Can you work these out from the model? Positions are in its coordinate system, mm. A direction names the side the tool comes from. Round coordinates to 2 decimals unless told otherwise and drop trailing zeros. Write each loop counter-clockwise with the first axis right and the second up, starting at its lowest first coordinate (ties: lowest second). Pieces come first, ordered by that corner, then holes. Notation, with made-up numbers: M 89.25,-34 L 103.25,-34 A17 ccw 103.25,-30 Z; hole C 45,36 d6. An arc over 180 degrees is marked long. Answer as a JSON object with one key per item and string values. Group by question number.
1) Please list where these lines run through material, in increasing order: L1, parallel to X at y = 14.75, z = 31; L2, parallel to X at y = 10.5, z = 2; L3, parallel to Z at x = -3, y = 12. Write a range as [from, to].
2) On a 3-axis mill with a long thin cutter (end or side, diameter ignored), from which of +Z, -Z, +X, -X, +Y, -Y can I reach the whole of each face in a straight line? I mean faces 4 (the flat face through (-4, 12, -37.5)), 5 (the flat face through (0, 13, 13.5)), 6 (the flat face through (-2, 13, 30)), 7 (the flat face through (3, 13, -31)). Say none if no direction works.
3) Suppose I cut it at A-A, the plane z = -29. Write out the boundary of the cut face in (x, y), and give its area (3 significant figures).
4) If we mould it in two halves opening along X, with no side actions, what happens to faces 1 (the flat face through (6, 12, 37.5)), 2 (the flat face through (9, 12, 1)), 3 (the flat face through (3, 13, 31))? For each: +X half, -X half, draft (parallel to the pull), parting line (faces both ways), or undercut.
5) Suppose I cut it at D-D, the plane y = 12.5. State how many separate pieces and enclosed holes the cut face has, and give its area (3 significant figures).
6) Suppose I cut it at C-C, the plane x = 4.25. Write out the boundary of the cut face in (y, z), and give its area (3 significant figures).
7) Suppose I cut it at B-B, the plane y = 9.5. Write out the boundary of the cut face in (x, z) (3 decimals), and give its area (3 significant figures).
8) I'm going to push flat-ended pins straight in: pin 1 Ø1.8 at (y, z) = (12.5, 32.62) entering from -X; pin 2 Ø3 at (y, z) = (6.5, -32.5) entering from -X; pin 3 Ø8.5 at (y, z) = (14, -31.5) entering from -X. Where does each tip first touch, or does it pass through?
Autodesk Inventor part; units mm, degrees
ref_plane "YZ Plane" through (0, 0, 0) normal (1, 0, 0) x (0, 1, 0)
ref_plane "XZ Plane" through (0, 0, 0) normal (0, 1, 0) x (-1, 0, 0)
ref_plane "XY Plane" through (0, 0, 0) normal (0, 0, 1) x (1, 0, 0)
sketch "Boceto2" plane through (0, 0, 0) normal (0, 1, 0) x (-1, 0, 0)
  line L0 (-10, 37.5) -> (10, 37.5)
  line L1 (10, 37.5) -> (10, -37.5)
  line L2 (10, -37.5) -> (-10, -37.5)
  line L3 (-10, -37.5) -> (-10, 37.5)
  line L4 (-10, 37.5) -> (10, -37.5) construction
  line L5 (10, 37.5) -> (-10, -37.5) construction
  point P0 (0, 0)
  dimension "d10" = 20
  dimension "d11" = 75
extrude "Extrusión1" add sketch "Boceto2" along normal blind 25
sketch "Boceto3" plane through (0, 25, 0) normal (0, 1, 0) x (1, 0, 0)
  line L0 (-10, -37.5) -> (10, -37.5)
  line L1 (10, -37.5) -> (10, 37.5)
  line L2 (10, 37.5) -> (-10, 37.5)
  line L3 (-10, 37.5) -> (-10, -37.5)
  arc A0 (3, -26.6962) -> (-2, -27.1569) centre (0, -21.5) ccw
  arc A1 (-8, -21.5) -> (-5, -27.745) centre (0, -21.5) ccw
  line L4 (-10, -37.5) -> (10, -37.5)
  line L5 (3, -37.5) -> (-2, -37.5)
  line L6 (3, -26.6962) -> (3, -37.5)
  line L7 (-5, -37.5) -> (-5, -27.745)
  line L8 (-8, -21.5) -> (-8, 21.5)
  line L9 (-5, -13.5) -> (5, -13.5)
  line L10 (-5, -13.5) -> (-5, 13.5)
  line L11 (7, 0) -> (10, 0)
  line L12 (-2, -37.5) -> (-2, -27.1569)
  line L13 (10, 0) -> (7, 0)
  arc A2 (-2, 27.1569) -> (3, 26.6962) centre (0, 21.5) ccw
  arc A3 (-5, 27.745) -> (-8, 21.5) centre (0, 21.5) ccw
  line L14 (3, 37.5) -> (-2, 37.5)
  line L15 (3, 26.6962) -> (3, 37.5)
  line L16 (-5, 37.5) -> (-5, 27.745)
  line L17 (-8, 21.5) -> (-8, 10)
  line L18 (-5, 13.5) -> (5, 13.5)
  line L19 (-5, 13.5) -> (-5, 10)
  line L20 (-2, 37.5) -> (-2, 27.1569)
  line L21 (5, -13.5) -> (5, 13.5)
  line L22 (-5, -37.5) -> (-10, -37.5)
  line L23 (-10, -37.5) -> (-10, 37.5)
  line L24 (10, 37.5) -> (-10, 37.5)
  line L25 (-10, 37.5) -> (-5, 37.5)
  point P0 (0, 0)
  point P1 (-8, -10)
  point P2 (-5, -10)
  dimension "d15" = 0
  dimension "d16" = 21.5
  dimension "d27" = 5
  dimension "d30" = 3
  dimension "d54" = 2
  dimension "d55" = 5
  dimension "d56" = 6
  dimension "d57" = 2
  dimension "d58" = 7
  dimension "d59" = 10
extrude "Extrusión3" cut sketch "Boceto3" against normal through all contours L12 A0 L6 L0 | L2 L15 A2 L20
extrude "Extrusión5" cut sketch "Boceto3" against normal through all contours L3 L2 L16 A3 L8 A1 L7 L0 | L10 L18 L21 L9
sketch "Boceto4" plane through (-8, 25, -21.5) normal (-1, 0, 0) x (0, 0, 1)
  line L0 (59, -25) -> (49.245, -25)
  line L1 (59, 0) -> (59, -25)
  line L2 (49.245, 0) -> (59, 0)
  line L3 (49.245, 0) -> (49.245, -25)
  line L4 (43, -25) -> (0, -25)
  line L5 (43, 0) -> (43, -25)
  line L6 (0, 0) -> (43, 0)
  line L7 (0, 0) -> (0, -25)
  line L8 (21.5, 0) -> (21.5, -25)
  line L9 (54.1225, -25) -> (54.1225, 0)
  line L10 (59, -12.5) -> (49.245, -12.5)
  point P0 (54.1225, -12.5)
  point P1 (54.1225, -12.5)
  point P2 (-11.1225, -12.5)
hole "Agujero1" at (-8, 12.5, 32.6225) at (-8, 12.5, -32.6225) direction (1, 0, 0) diameter 3 end through all
sketch "Boceto5" plane through (0, 0, 0) normal (0, -1, 0) x (1, 0, 0)
  line L0 (-5, -27.745) -> (-5, -37.5)
  line L1 (-5, -37.5) -> (-2, -37.5)
  line L2 (-2, -37.5) -> (-2, -27.1569)
  arc A0 (3, -26.6962) -> (-2, -27.1569) centre (0, -21.5) ccw
  line L3 (3, -26.6962) -> (3, -37.5)
  line L4 (3, -37.5) -> (10, -37.5)
  line L5 (10, -37.5) -> (10, 37.5)
  line L6 (10, 37.5) -> (3, 37.5)
  line L7 (3, 37.5) -> (3, 26.6962)
  arc A1 (-2, 27.1569) -> (3, 26.6962) centre (0, 21.5) ccw
  line L8 (-2, 27.1569) -> (-2, 37.5)
  line L9 (-2, 37.5) -> (-5, 37.5)
  line L10 (-5, 37.5) -> (-5, 27.745)
  arc A2 (-5, 27.745) -> (-8, 21.5) centre (0, 21.5) ccw
  line L11 (-8, 21.5) -> (-8, -21.5)
  arc A3 (-8, -21.5) -> (-5, -27.745) centre (0, -21.5) ccw
  line L12 (5, 13.5) -> (5, -13.5)
  line L13 (5, -13.5) -> (-5, -13.5)
  line L14 (-5, -13.5) -> (-5, 13.5)
  line L15 (-5, 13.5) -> (5, 13.5)
  line L16 (6, -21.5) -> (6, 21.5)
  arc A4 (-2, 27.1569) -> (3, 26.6962) centre (0, 21.5) ccw
  arc A5 (3, -26.6962) -> (-2, -27.1569) centre (0, -21.5) ccw
  line L17 (9, 37.5) -> (9, -37.5)
  point P0 (0, 0)
  dimension "d60" = 3
extrude "Extrusión6" cut sketch "Boceto5" against normal through all contours L17 L6 L5 L4
equation "\"d10\" = 20 * scale"
equation "\"d11\" = 75 * scale"
equation "\"d12\" = 25 * scale"
equation "\"d27\" = 5 * scale"
equation "\"d30\" = 3 * scale"
equation "\"d54\" = 2 * scale"
equation "\"d55\" = 5 * scale"
equation "\"d56\" = 6 * scale"
equation "\"d57\" = 2 * scale"
equation "\"d58\" = 7 * scale"
equation "\"d59\" = 10 * scale"
equation "\"scale\" = 1"
properties part number "PiezaPeluda"
Results:
{
 "1": {"L1": "[-5, -2], [3, 9]", "L2": "[-8, -5], [5, 9]", "L3": "[-37.5, -34.04], [-31.21, -26.7], [-16.3, -13.5], [13.5, 16.3], [26.7, 31.21], [34.04, 37.5]"},
 "2": {"face 4": "-Z, +X, -X, +Y, -Y", "face 5": "+Y, -Y", "face 6": "+Z, +Y, -Y", "face 7": "-Z, +Y, -Y"},
 "3": {"outline": "M -5,0 L -2,0 L -2,25 L -5,25 Z; M 3,0 L 9,0 L 9,25 L 3,25 Z", "area": "225 mm^2"},
 "4": {"face 1": "draft", "face 2": "+X half", "face 3": "undercut"},
 "5": {"separate pieces": "5", "enclosed holes": "1", "area": "553 mm^2"},
 "6": {"outline": "M 0,-37.5 L 25,-37.5 L 25,-25.74 L 0,-25.74 Z; M 0,-17.26 L 25,-17.26 L 25,-13.5 L 0,-13.5 Z; M 0,13.5 L 25,13.5 L 25,17.26 L 0,17.26 Z; M 0,25.74 L 25,25.74 L 25,37.5 L 0,37.5 Z; hole C 12.5,-32.62 d3; hole C 12.5,32.62 d3", "area": "762 mm^2"},
 "7": {"outline": "M -8,-21.5 A8 ccw -5,-27.745 L -5,-37.5 L -2,-37.5 L -2,-27.157 A6 cw long 3,-26.696 L 3,-37.5 L 9,-37.5 L 9,37.5 L 3,37.5 L 3,26.696 A6 cw long -2,27.157 L -2,37.5 L -5,37.5 L -5,27.745 A8 ccw -8,21.5 Z; hole M -5,-13.5 L 5,-13.5 L 5,13.5 L -5,13.5 Z", "area": "607 mm^2"},
 "8": {"pin 1": "through", "pin 2": "x = -5", "pin 3": "x = -5.56"}
}
